Source: CAD feature listing. Evaluate the final solid. Frame: model axes, mm. Face numbers are marked on the shaded views. Coordinates: 2 decimals unless noted, no trailing zeros. Order: outer loops, then holes, each group sorted by start corner. A loop starts at its lowest first (then second) coordinate and runs counter-clockwise, first axis right, second up.
Item 1: Section D-D on x = -72.5. Return the cut outline in (y, z).
Item 2: Contact query for flat-ended pins moving along their axis: P1, Ø2, axis at y = 21.5, z = 7.5, coming from the +X side; P2, Ø2, axis at y = 192.5, z = 2, coming from the +X side; P3, Ø3, axis at x = 28.5, z = 8.5, coming from the -Y side. Output: stop coordinate, or through.
Item 3: Section B-B on z = 9.75. Return the cut outline in (x, y), then the cut area to 3 significant figures.
Item 4: Mould query, pull axis Y, two halves, no side actions, for the marked faces 1 and 2. Classes: released by +Y, released by -Y, zero draft, split by the parting line, or undercut.
Item 5: Section C-C on y = -5.5. Return the cut outline in (x, z), then the cut area to 3 significant figures.
Item 6: Ray query, line 1 (Y direction, x = 0, z = 5.75); line 2 (X direction, y = 117, z = 2); line 3 (X direction, y = -17.5, z = 10.75). Return the intervals inside material, ascending.
Item 7: Section A-A on x = 0. Return the cut outline in (y, z), then the cut area to 3 significant figures.
from build123d import *

# Parameters (mm, degrees)
SKETCH_1_R      = 37.5
EXTRUDE_1_DEPTH = 12
FILLET_1_R      = 10
FILLET_2_R      = 30


with BuildPart() as part:
    # 草图1 → 凸台-拉伸1 (new body)
    with BuildSketch(Plane.XY):
        with BuildLine():
            Line((-42.858365035, -25.751903746), (-100, 69.347746915))
            Line((-100, 69.347746915), (-100, 160))
            Line((-100, 160), (-70, 220))
            Line((-70, 220), (-25, 220))
            Line((-25, 220), (-25, 100))
            Line((-25, 100), (39.764990452, 100))
            Line((39.764990452, 100), (49.726094768, 5.226423163))
            ThreePointArc((49.726094768, 5.226423163), (15.86523282, -47.41618276), (-42.858365035, -25.751903746))
        make_face()
        Circle(SKETCH_1_R, mode=Mode.SUBTRACT)
    extrude(amount=EXTRUDE_1_DEPTH)

    # 圆角1
    fillet_1_edges = [part.edges().sort_by_distance(p)[0] for p in [
        (-25, 220, 6),
        (39.764990452, 100, 6),
    ]]
    fillet(fillet_1_edges, radius=FILLET_1_R)

    # 圆角2
    fillet_2_edges = [part.edges().sort_by_distance(p)[0] for p in [
        (-100, 69.347746915, 6),
        (-100, 160, 6),
    ]]
    fillet(fillet_2_edges, radius=FILLET_2_R)


solid = part.part
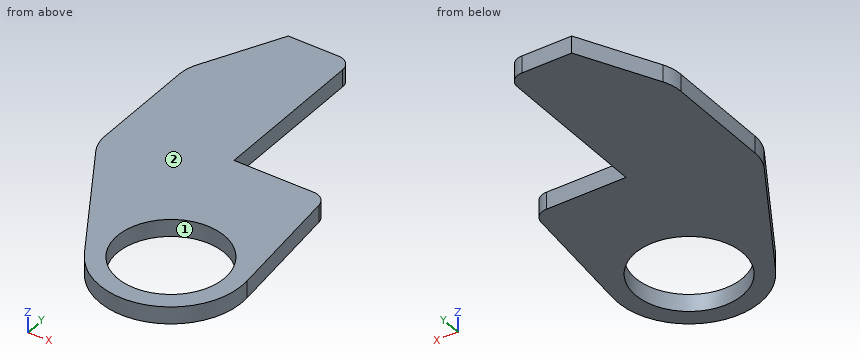
Answer list:
1. outline: (23.58, 0) - (215, 0) - (215, 12) - (23.58, 12) - close
2. P1: stops at x = 48.12
2. P2: stops at x = -25
2. P3: stops at y = -42.08
3. outline: (-100, 77.67) arc R30 ccw to (-95.72, 62.22) - (-42.86, -25.75) arc R50 ccw to (49.73, 5.23) - (40.71, 91.05) arc R10 ccw to (30.76, 100) - (-25, 100) - (-25, 210) arc R10 ccw to (-35, 220) - (-70, 220) - (-96.83, 166.33) arc R30 ccw to (-100, 152.92) - close; hole circle Ø75 at (0, 0)
3. area: 20,700 mm2
4. face 1: undercut
4. face 2: zero draft
5. outline: (-55.03, 0) - (-37.09, 0) - (-37.09, 12) - (-55.03, 12) - close; (37.09, 0) - (49.7, 0) - (49.7, 12) - (37.09, 12) - close
5. area: 366 mm2
6. line 1: y = -50 to -37.5, 37.5 to 100
6. line 2: x = -100 to -25
6. line 3: x = -47.82 to -33.17, 33.17 to 46.84
7. outline: (-50, 0) - (-37.5, 0) - (-37.5, 12) - (-50, 12) - close; (37.5, 0) - (100, 0) - (100, 12) - (37.5, 12) - close
7. area: 900 mm2
